Geometry: final body of the model. Coordinates: model frame, mm. A direction names the side the tool comes from. Coordinates: 2 decimals unless noted, no trailing zeros. Write each loop counter-clockwise with the first axis right and the second up, starting at its lowest first coordinate (ties: lowest second). Pieces come first, ordered by that corner, then holes. Notation, with made-up numbers: M -3.75,66.5 L 48.25,66.5 A21 cw 48.25,84.5 Z; hole C 85.5,-39.75 d4. An arc over 180 degrees is marked long. Write item = value, one per line. Start each with the question number.
Item 1: Ray query, L1, parallel to X at y = 38, z = 9.25; L2, parallel to Y at x = 16.5, z = 6.5; L3, parallel to Y at x = 6.5, z = 9. Return the intervals inside material, ascending. Write a range as [from, to].
Item 2: Section B-B on x = 37. Output: boundary loops of the cut face in (y, z), plus the area to 3 significant figures.
Item 3: Section C-C on y = 23. Output: boundary loops of the cut face in (x, z), plus the area to 3 significant figures.
Item 4: Pull-direction query (X, two-part tool) for faces 4 (the cylindrical face through (1.141, 1.203, 4.056)), 5 (the flat face through (50, 52, 4)), 6 (the flat face through (59, 1, 6.5)); classes: +X half, -X half, draft (parallel to the pull), parting line (faces both ways), or undercut.
Item 5: First-contact query: pin 1 Ø1.2 at (x, y) = (66, 1.5) entering from +Z; pin 2 Ø4 at (x, y) = (16, 21) entering from -Z; pin 3 Ø5 at (x, y) = (12.5, 9.5) entering from +Z; pin 4 Ø1.2 at (y, z) = (1, 7.5) entering from -X. Flat tips, straight axial feed; report the tip coordinate or a pass-through.
Item 6: Section A-A on z = 5. Output: boundary loops of the cut face in (x, y), plus the area to 3 significant figures.
Item 7: Reachability of faces 1 (the flat face through (99.5, 26, 5)), 2 (the cylindrical face through (99.959, 49.176, 9.019)), 3 (the cylindrical face through (2.08, 2.77, 9.02)) from +Z, -Z, +X, -X, +Y, -Y: full face, straight path, thin tool, end or side. Return the list, or none.
from build123d import *

# Parameters (mm, degrees)
ESQUISSE1_W             = 102
ESQUISSE1_H             = 52
BOSS_EXTRU_1_DEPTH      = 2
ESQUISSE2_W             = 102
ESQUISSE2_H             = 52
ESQUISSE2_W_2           = 97
ESQUISSE2_H_2           = 47
EXTRU_MINCE1_DEPTH      = 6
CONG_2_R                = 4
ESQUISSE4_W             = 42
ESQUISSE4_H             = 22.824396381
ENL_V_MAT_EXTRU_1_DEPTH = 14
EXTRU_MINCE2_DEPTH      = 2
EXTRU_MINCE2_DRAFT      = 1
CONG_3_R                = 3


with BuildPart() as part:
    # Esquisse1 → Boss.-Extru.1 (new body)
    with BuildSketch(Plane.XY):
        with Locations((51, 26)):
            Rectangle(ESQUISSE1_W, ESQUISSE1_H)
    extrude(amount=BOSS_EXTRU_1_DEPTH)

    # Esquisse2 → Extru.-Mince1 (add)
    with BuildSketch(Plane.XY.offset(2)):
        with Locations((51, 26)):
            Rectangle(ESQUISSE2_W, ESQUISSE2_H)
        with Locations((51, 26)):
            Rectangle(ESQUISSE2_W_2, ESQUISSE2_H_2, mode=Mode.SUBTRACT)
    extrude(amount=EXTRU_MINCE1_DEPTH)

    # Congé2
    cong_2_edges = [part.edges().sort_by_distance(p)[0] for p in [
        (0, 52, 4),
        (102, 52, 4),
        (102, 0, 4),
        (0, 0, 4),
    ]]
    fillet(cong_2_edges, radius=CONG_2_R)

    # Esquisse4 → Enlèv. mat.-Extru.1 (cut)
    with BuildSketch(Plane(origin=(0, 0, 0), x_dir=(1, 0, 0), z_dir=(0, 1, 0))):
        with Locations((59, -17.91219819)):
            Rectangle(ESQUISSE4_W, ESQUISSE4_H)
    extrude(amount=ENL_V_MAT_EXTRU_1_DEPTH, mode=Mode.SUBTRACT)


with BuildPart() as extru_mince2_tool:
    # Esquisse5 → Extru.-Mince2 (with draft: the straight prism first)
    with BuildSketch(Plane.XY.offset(8)):
        Polygon((38, 2.5), (2.5, 2.5), (2.5, 49.5), (99.5, 49.5), (99.5, 2.5), (80, 2.5), (80, 1.5), (100.5, 1.5), (100.5, 50.5), (1.5, 50.5), (1.5, 1.5), (38, 1.5), align=None)
    extrude(amount=EXTRU_MINCE2_DEPTH)
    # Extru.-Mince2: the draft: its side faces are tilted about the plane it starts from
    extru_mince2_sides = [extru_mince2_tool.faces().sort_by_distance(p)[0] for p in [
        (20.25, 2.5, 9),
        (2.5, 26, 9),
        (51, 49.5, 9),
        (99.5, 26, 9),
        (89.75, 2.5, 9),
        (80, 2, 9),
        (90.25, 1.5, 9),
        (100.5, 26, 9),
        (51, 50.5, 9),
        (1.5, 26, 9),
        (19.75, 1.5, 9),
        (38, 2, 9),
    ]]
    draft(extru_mince2_sides, Plane.XY.offset(8), EXTRU_MINCE2_DRAFT)


with BuildPart() as part_1:
    add(part.part)

    # Extru.-Mince2: add extru_mince2_tool
    add(extru_mince2_tool.part)

    # Congé3
    cong_3_edges = [part_1.edges().sort_by_distance(p)[0] for p in [
        (100.482544935, 1.517455065, 9),
        (100.482544935, 50.482544935, 9),
        (1.517455065, 50.482544935, 9),
        (1.517455065, 1.517455065, 9),
    ]]
    fillet(cong_3_edges, radius=CONG_3_R)


solid = part_1.part
Responses:
q1.L1 = [1.52, 2.48], [99.52, 100.48]
q1.L2 = [0, 2.5], [49.5, 52]
q1.L3 = [1.52, 2.48], [49.52, 50.48]
q2.outline = M 0,0 L 52,0 L 52,8 L 50.5,8 L 50.47,10 L 49.53,10 L 49.5,8 L 49.5,2 L 2.5,2 L 2.5,8 L 2.47,10 L 1.53,10 L 1.5,8 L 0,8 Z
q2.area = 138 mm²
q3.outline = M 0,0 L 102,0 L 102,8 L 100.5,8 L 100.47,10 L 99.53,10 L 99.5,8 L 99.5,2 L 2.5,2 L 2.5,8 L 2.47,10 L 1.53,10 L 1.5,8 L 0,8 Z
q3.area = 238 mm²
q4.face_4 = -X half
q4.face_5 = draft
q4.face_6 = undercut
q5.pin_1 = 6.5
q5.pin_2 = 0
q5.pin_3 = 2
q5.pin_4 = 0.8
q6.outline = M 0,4 A4 ccw 4,0 L 98,0 A4 ccw 102,4 L 102,48 A4 ccw 98,52 L 4,52 A4 ccw 0,48 Z; hole M 2.5,2.5 L 99.5,2.5 L 99.5,49.5 L 2.5,49.5 Z
q6.area = 731 mm²
q7.face_1 = +Z
q7.face_2 = +Z, +X, +Y
q7.face_3 = +Z, -X, -Y
